from build123d import *

# Parameters (mm, degrees)
SKETCH_1_W      = 50
SKETCH_1_H      = 16.25
SKETCH_1_R      = 2.5
EXTRUDE_1_DEPTH = 1.2
SKETCH_2_R      = 1.005653766
EXTRUDE_2_DEPTH = 50


with BuildPart() as part:
    # 草图1 → 凸台-拉伸1 (new body)
    with BuildSketch(Plane(origin=(0, 0, 0), x_dir=(1, 0, 0), z_dir=(0, 1, 0))):
        with Locations((25, -8.125)):
            Rectangle(SKETCH_1_W, SKETCH_1_H)
        with Locations(Location((7, -8.5, 0), (0, 0, 270))):
            Circle(SKETCH_1_R, mode=Mode.SUBTRACT)
        with Locations(Location((43, -8.5, 0), (0, 0, 270))):
            Circle(SKETCH_1_R, mode=Mode.SUBTRACT)
        with Locations(Location((25, -11.25, 0), (0, 0, 270))):
            Circle(SKETCH_1_R, mode=Mode.SUBTRACT)
    extrude(amount=EXTRUDE_1_DEPTH)

    # 草图2 → 凸台-拉伸2 (add)
    with BuildSketch(Plane.ZY):
        with BuildLine():
            Line((0, 0), (-3.25, 0))
            ThreePointArc((-3.25, 0), (-5.548097039, 5.548097039), (0, 3.25))
            Line((0, 3.25), (0, 0))
        make_face()
        with Locations((-3.25, 3.25)):
            Circle(SKETCH_2_R, mode=Mode.SUBTRACT)
    extrude(amount=-EXTRUDE_2_DEPTH)


solid = part.part
Could you check a few things on this model? Use its own coordinates, in mm. A direction names the side the tool comes from. Give positions to 0.01 mm unless a question says otherwise; leave off trailing zeros. Order: outer loops, then holes, each group sorted by start corner. A loop starts at its lowest first (then second) coordinate and runs counter-clockwise, first axis right, second up. Notation, with made-up numbers: (29, -8) - (52, -8) arc R5 ccw to (52, -2) - close; hole circle Ø1 at (8.25, 48.25). An arc over 180 degrees is marked (long way). One line per item, written item: value. Start each with the question number.
1. For P1, Ø3, axis at x = 29, z = 14, coming from the +Y side; P2, Ø1.8, axis at y = 3.25, z = -3.25, coming from the +X side; P3, Ø2.5, axis at x = 24.5, y = 2.5, coming from the +Z side; P4, Ø3, axis at y = 1.5, z = 6, coming from the -X side, each with a flat end and sliding along its axis, tell me the tip position at first contact or that it passes through.
2. Imagine slicing it at A-A on x = 7. List the corners of the cut face in (y, z) for me, plus the area to 3 significant figures.
3. Thinking about a two-plate mould opening in X: for faces 3 (the face through (5, 1, 10)), 4 (the face through (0, 1, 3)), 5 (the face through (24.65, 5.471, -5.623)), which applies, +X half, -X half, draft (parallel to the pull), parting line (faces both ways), or undercut?
4. If I drill on probe 1 along X at (y, z) = (0.7, 8.5); probe 2 along X at (y, z) = (0.6, 11.25); probe 3 along Y at (x, z) = (32, -3.25), over which ranges is the centre line in solid material (lowest first)?
5. For faces 1 (the face through (25, 1.2, 8)), 2 (the face through (27.48, 0.59, 10.92)), which set-ups out of +Z, -Z, +X, -X, +Y, -Y let a thin tool reach every point of the face, with its end or its side?
6. Imagine slicing it at B-B on y = 5. List the corners of the cut face in (x, z) for me.
Values:
1. P1: y = 1.2
1. P2: through
1. P3: z = 0
1. P4: x = 0
2. outline: (0, -3.25) arc R3.25 ccw (long way) to (3.25, 0) - (1.2, 0) - (1.2, 6) - (0, 6) - close; (0, 11) - (1.2, 11) - (1.2, 16.25) - (0, 16.25) - close; hole circle Ø2.01 at (3.25, -3.25)
2. area: 45.8 mm²
3. face 3: undercut
3. face 4: -X half
3. face 5: draft
4. probe 1: 0 to 4.5, 9.5 to 40.5, 45.5 to 50
4. probe 2: 0 to 22.5, 27.5 to 50
4. probe 3: 0 to 2.24, 4.26 to 6.5
5. face 1: +Z, +X, -X, +Y
5. face 2: +Y, -Y
6. outline: (0, -5.99) - (50, -5.99) - (50, -0.51) - (0, -0.51) - close
